The model under review builds one solid part; all positions refer to its coordinate system, in mm. Round coordinates to 2 decimals unless told otherwise and drop trailing zeros. Loops run counter-clockwise (first coordinate to the right, second up) from the corner with the lowest first, then second, coordinate; pieces in that order, holes last. Notation, with made-up numbers: (19.25, 69) -> (40.25, 69) arc R29 ccw to (40.25, 101) -> close; hole circle Ø6 at (-22, -16). An arc over 180 degrees is marked (long way). Use a Markdown table: item, result. Add a question column.
1) Consider section C-C on x = -49. Give the boundary of the cut face in (y, z) (3 decimals).
2) Wall thickness on probe 1 along X at (y, z) = (154, 2.7) (3 decimals); probe 2 along Y at (x, z) = (0, 1) (3 decimals); probe 3 along Y at (x, z) = (21.5, 0.45): over which ranges is each line inside the solid? List them lowest first.
3) Insertion check: pin 1 (1.6 mm diameter, centred on y = 128.5, z = 1.5, fed in from -X) (3 decimals); pin 2 (1.8 mm diameter, centred on x = -55.56, y = 138.56, fed in from +Z); pin 3 (1.6 mm diameter, centred on y = -3, z = 1, fed in from +X) (3 decimals). Each pin has a flat end and moves straight along its axis. Give the tip position at first contact, or say it passes through.
4) Consider section D-D on y = 75. Give the boundary of the cut face in (x, z) (3 decimals).
5) Consider section A-A on y = 11.43. Give the boundary of the cut face in (x, z) (3 decimals).
6) Consider section B-B on x = 0. Give the boundary of the cut face in (y, z) (3 decimals), plus the area to 3 significant figures.
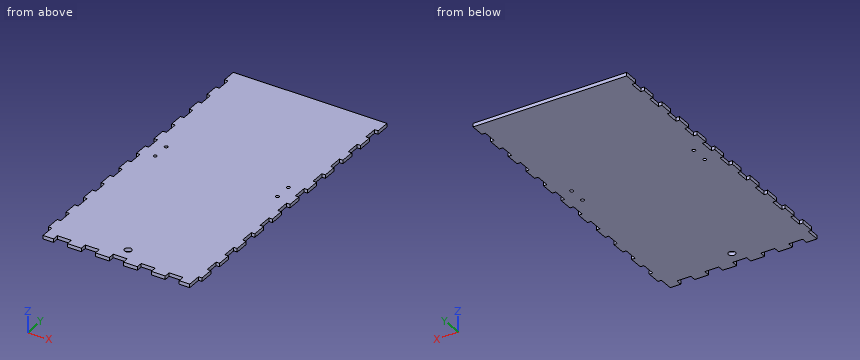
from build123d import *

# Parameters (mm, degrees)
SKETCH1_W           = 3.175
SKETCH1_H           = 12.7
SKETCH1_W_2         = 9.525
SKETCH1_H_2         = 5.588
SKETCH1_W_3         = 12.7
BOSS_EXTRUDE1_DEPTH = 3.175
SKETCH2_R           = 3.175
CUT_EXTRUDE1_DEPTH  = 4.175
SKETCH3_R           = 1.5
CUT_EXTRUDE2_DEPTH  = 4.175


with BuildPart() as part:
    # Sketch1 → Boss-Extrude1 (new body)
    with BuildSketch(Plane.XY):
        Polygon((-66.675, 273.812), (-66.675, 261.112), (-66.675, 248.412), (-66.675, 235.712), (-66.675, 223.012), (-66.675, 210.312), (-66.675, 197.612), (-66.675, 184.912), (-66.675, 172.212), (-66.675, 159.512), (-66.675, 146.812), (-66.675, 134.112), (-66.675, 121.412), (-66.675, 108.712), (-66.675, 96.012), (-66.675, 83.312), (-66.675, 70.612), (-66.675, 57.912), (-66.675, 45.212), (-66.675, 32.512), (-66.675, 19.812), (-66.675, 7.112), (-66.675, 0), (-57.15, 0), (-44.45, 0), (-31.75, 0), (-19.05, 0), (-6.35, 0), (6.35, 0), (19.05, 0), (31.75, 0), (44.45, 0), (57.15, 0), (66.675, 0), (66.675, 7.112), (66.675, 19.812), (66.675, 32.512), (66.675, 45.212), (66.675, 57.912), (66.675, 70.612), (66.675, 83.312), (66.675, 96.012), (66.675, 108.712), (66.675, 121.412), (66.675, 134.112), (66.675, 146.812), (66.675, 159.512), (66.675, 172.212), (66.675, 184.912), (66.675, 197.612), (66.675, 210.312), (66.675, 223.012), (66.675, 235.712), (66.675, 248.412), (66.675, 261.112), (66.675, 273.812), align=None)
        with Locations((-68.2625, 13.462)):
            Rectangle(SKETCH1_W, SKETCH1_H)
        with Locations((-68.2625, 38.862)):
            Rectangle(SKETCH1_W, SKETCH1_H)
        with Locations((-68.2625, 64.262)):
            Rectangle(SKETCH1_W, SKETCH1_H)
        with Locations((-68.2625, 89.662)):
            Rectangle(SKETCH1_W, SKETCH1_H)
        with Locations((-61.9125, -2.794)):
            Rectangle(SKETCH1_W_2, SKETCH1_H_2)
        with Locations((-38.1, -2.794)):
            Rectangle(SKETCH1_W_3, SKETCH1_H_2)
        with Locations((-12.7, -2.794)):
            Rectangle(SKETCH1_W_3, SKETCH1_H_2)
        with Locations((12.7, -2.794)):
            Rectangle(SKETCH1_W_3, SKETCH1_H_2)
        with Locations((38.1, -2.794)):
            Rectangle(SKETCH1_W_3, SKETCH1_H_2)
        with Locations((61.9125, -2.794)):
            Rectangle(SKETCH1_W_2, SKETCH1_H_2)
        with Locations((68.2625, 13.462)):
            Rectangle(SKETCH1_W, SKETCH1_H)
        with Locations((68.2625, 38.862)):
            Rectangle(SKETCH1_W, SKETCH1_H)
        with Locations((68.2625, 64.262)):
            Rectangle(SKETCH1_W, SKETCH1_H)
        with Locations((68.2625, 89.662)):
            Rectangle(SKETCH1_W, SKETCH1_H)
        with Locations((68.2625, 115.062)):
            Rectangle(SKETCH1_W, SKETCH1_H)
        with Locations((-68.2625, 115.062)):
            Rectangle(SKETCH1_W, SKETCH1_H)
        with Locations((-68.2625, 140.462)):
            Rectangle(SKETCH1_W, SKETCH1_H)
        with Locations((-68.2625, 165.862)):
            Rectangle(SKETCH1_W, SKETCH1_H)
        with Locations((-68.2625, 191.262)):
            Rectangle(SKETCH1_W, SKETCH1_H)
        with Locations((-68.2625, 216.662)):
            Rectangle(SKETCH1_W, SKETCH1_H)
        with Locations((-68.2625, 242.062)):
            Rectangle(SKETCH1_W, SKETCH1_H)
        with Locations((-68.2625, 267.462)):
            Rectangle(SKETCH1_W, SKETCH1_H)
        with Locations((68.2625, 140.462)):
            Rectangle(SKETCH1_W, SKETCH1_H)
        with Locations((68.2625, 165.862)):
            Rectangle(SKETCH1_W, SKETCH1_H)
        with Locations((68.2625, 191.262)):
            Rectangle(SKETCH1_W, SKETCH1_H)
        with Locations((68.2625, 216.662)):
            Rectangle(SKETCH1_W, SKETCH1_H)
        with Locations((68.2625, 242.062)):
            Rectangle(SKETCH1_W, SKETCH1_H)
        with Locations((68.2625, 267.462)):
            Rectangle(SKETCH1_W, SKETCH1_H)
    extrude(amount=BOSS_EXTRUDE1_DEPTH)

    # Sketch2 → Cut-Extrude1 (cut, through all)
    with BuildSketch(Plane.XY.offset(3.175)):
        with Locations((0, 11.43)):
            Circle(SKETCH2_R)
    extrude(amount=-CUT_EXTRUDE1_DEPTH, mode=Mode.SUBTRACT)

    # Sketch3 → Cut-Extrude2 (cut, through all)
    with BuildSketch(Plane.XY.offset(3.175)):
        with Locations((-55.5625, 154.305)):
            Circle(SKETCH3_R)
        with Locations((-55.5625, 138.557)):
            Circle(SKETCH3_R)
        with Locations((55.5625, 154.305)):
            Circle(SKETCH3_R)
        with Locations((55.5625, 138.557)):
            Circle(SKETCH3_R)
    extrude(amount=-CUT_EXTRUDE2_DEPTH, mode=Mode.SUBTRACT)


solid = part.part
Result set:
| question | item | result |
|---|---|---|
| 1 | outline | (0, 0) -> (273.812, 0) -> (273.812, 3.175) -> (0, 3.175) -> close |
| 2 | probe 1 | -66.675 to -57.031, -54.094 to 54.094, 57.031 to 66.675 |
| 2 | probe 2 | 0 to 8.255, 14.605 to 273.812 |
| 2 | probe 3 | 0 to 273.81 |
| 3 | pin 1 | x = -66.675 |
| 3 | pin 2 | through |
| 3 | pin 3 | x = 66.675 |
| 4 | outline | (-66.675, 0) -> (66.675, 0) -> (66.675, 3.175) -> (-66.675, 3.175) -> close |
| 5 | outline | (-69.85, 0) -> (-3.175, 0) -> (-3.175, 3.175) -> (-69.85, 3.175) -> close; (3.175, 0) -> (69.85, 0) -> (69.85, 3.175) -> (3.175, 3.175) -> close |
| 6 | outline | (0, 0) -> (8.255, 0) -> (8.255, 3.175) -> (0, 3.175) -> close; (14.605, 0) -> (273.812, 0) -> (273.812, 3.175) -> (14.605, 3.175) -> close |
| 6 | area | 849 mm2 |
